Design review of the part built by this model. Coordinates are the model's own, in mm. Face numbers are marked on the shaded views. A direction names the side the tool comes from. Give positions to 0.01 mm unless a question says otherwise; leave off trailing zeros. Loops run counter-clockwise (first coordinate to the right, second up) from the corner with the lowest first, then second, coordinate; pieces in that order, holes last.
Autodesk Inventor part; units mm, degrees
ref_plane "YZ Plane" through (0, 0, 0) normal (1, 0, 0) x (0, 1, 0)
ref_plane "XZ Plane" through (0, 0, 0) normal (0, 1, 0) x (-1, 0, 0)
ref_plane "XY Plane" through (0, 0, 0) normal (0, 0, 1) x (1, 0, 0)
sketch "Sketch8" plane through (0, 0, 0) normal (0, 1, 0) x (-1, 0, 0)
  line L0 (-13.5, -17.5) -> (13.5, -17.5)
  line L1 (13.5, -17.5) -> (13.5, 17.5)
  line L2 (13.5, 17.5) -> (-13.5, 17.5)
  line L3 (-13.5, 17.5) -> (-13.5, -17.5)
  line L4 (-13.5, -17.5) -> (13.5, 17.5) construction
  line L5 (13.5, -17.5) -> (-13.5, 17.5) construction
  circle A0 centre (10, -7.5) radius 1.6
  circle A1 centre (10, 7.5) radius 1.6
  circle A2 centre (-10, 7.5) radius 1.6
  circle A3 centre (-10, -7.5) radius 1.6
  point P0 (0, 0)
  dimension "d38" = 35
  dimension "d39" = 27
  dimension "d40" = 20
  dimension "d41" = 15
  dimension "d42" = 7.5
  dimension "d43" = 10
  dimension "d44" = 3.2
extrude "Extrusion7" add sketch "Sketch8" against normal blind 3
sketch "Sketch14" plane through (0, 0, 0) normal (0, 1, 0) x (1, 0, 0)
  line L0 (-13.5, 17.5) -> (-13.5, -17.5)
  line L1 (-13.5, -17.5) -> (13.5, -17.5)
  line L2 (13.5, -17.5) -> (13.5, 17.5)
  line L3 (13.5, 17.5) -> (-13.5, 17.5)
  circle A0 centre (-10, 7.5) radius 1.6
  circle A1 centre (-10, -7.5) radius 1.6
  circle A2 centre (10, -7.5) radius 1.6
  circle A3 centre (10, 7.5) radius 1.6
  line L4 (13.5, -17.5) -> (13.5, 17.5)
  line L5 (13.5, 4.5) -> (7.5, 4.5)
  line L6 (7.5, 4.5) -> (7.5, -4.5)
  line L7 (7.5, -4.5) -> (13.5, -4.5)
  line L8 (13.5, -4.5) -> (13.5, 4.5)
  point P0 (0, 0)
  dimension "d79" = 7.5
  dimension "d80" = 3
  dimension "d81" = 3
extrude "Extrusion12" add sketch "Sketch14" along normal blind 22.3 contours L2 L7 L6 L5
sketch "Sketch15" plane through (13.5, -3, 17.5) normal (1, 0, 0) x (0, 0, -1)
  line L0 (0, 3) -> (13, 3)
  line L1 (0, 3) -> (0, 0)
  line L2 (35, 0) -> (0, 0)
  line L3 (35, 3) -> (35, 0)
  line L4 (22, 3) -> (35, 3)
  line L5 (22, 3) -> (22, 25.3)
  line L6 (13, 25.3) -> (22, 25.3)
  line L7 (13, 3) -> (13, 25.3)
  line L8 (35, 3) -> (35, 0)
  line L9 (35, 0) -> (41.8017, 14.6399)
  circle A0 centre (35, 17.8) radius 2.6
  circle A1 centre (35, 17.8) radius 7.5
  circle A2 centre (0, 17.8) radius 2.6
  circle A3 centre (0, 17.8) radius 7.5
  line L10 (-275, -9) -> (225, -9)
  line L11 (0, 0) -> (-6.8017, 14.6399)
  line L12 (0, 25.3) -> (35, 25.3)
  point P0 (17.5, 3)
  point P1 (13, 25.3)
  point P2 (22, 25.3)
  dimension "d84" = 5.2
  dimension "d85" = 35
  dimension "d86" = 17.5
  dimension "d87" = 26.8
  dimension "d88" = 15
extrude "Extrusion13" add sketch "Sketch15" against normal blind 3 contours L1 L11 A3 L12 L7 L0 | L3 L4 L5 L12 A1 L9 | A3 | A1
sketch "Sketch16" plane through (10.5, -3, 17.5) normal (-1, 0, 0) x (0, 0, 1)
  arc A0 (-35, 25.3) -> (-41.8017, 14.6399) centre (-35, 17.8) ccw
  line L0 (-41.8017, 14.6399) -> (-35, 0)
  line L1 (-35, 3) -> (-35, 0)
  line L2 (-26.5199, 3) -> (-35, 3)
  line L3 (-26.5199, 3) -> (-23.4801, 3)
  line L4 (-22, 3) -> (-23.4801, 3)
  line L5 (-22, 25.3) -> (-22, 3)
  line L6 (-22, 25.3) -> (-35, 25.3)
  circle A1 centre (-35, 17.8) radius 2.6
  arc A2 (6.8017, 14.6399) -> (0, 25.3) centre (0, 17.8) ccw
  line L7 (0, 25.3) -> (-13, 25.3)
  line L8 (-13, 3) -> (-13, 25.3)
  line L9 (-11.5199, 3) -> (-13, 3)
  line L10 (-11.5199, 3) -> (-8.4801, 3)
  line L11 (0, 3) -> (-8.4801, 3)
  line L12 (0, 0) -> (0, 3)
  line L13 (0, 0) -> (6.8017, 14.6399)
  circle A3 centre (0, 17.8) radius 2.6
  line L14 (-22, 3) -> (-29, 3)
  line L15 (-29, 3) -> (-29, 13)
  line L16 (-29, 13) -> (-22, 13)
  line L17 (-22, 13) -> (-22, 3)
  line L18 (-11.5199, 3) -> (-13, 3)
  line L19 (-13, 3) -> (-6, 3)
  line L20 (-6, 3) -> (-6, 13)
  line L21 (-6, 13) -> (-13, 13)
  line L22 (-13, 13) -> (-13, 3)
  line L23 (-23.4, 0) -> (-26.6, 0)
  line L24 (-26.6, 3) -> (-23.4, 3)
  line L25 (-8.4, 0) -> (-11.6, 0)
  line L26 (-11.6, 3) -> (-8.4, 3)
  point P0 (-17.5, 3)
  point P1 (-10, 0)
  point P2 (-6, 3)
  dimension "d91" = 7
  dimension "d92" = 3
  dimension "d93" = 10
extrude "Extrusion14" cut sketch "Sketch16" against normal blind 22.3 contours L5 L4 L3 L2 L15 L16 | L21 L20 L11 L10 L9 L8
sketch "Sketch17" plane through (10.5, -3, 17.5) normal (-1, 0, 0) x (0, 0, 1)
  circle A0 centre (-35, 17.8) radius 2.6
  line L0 (-29, 3) -> (-29, 13)
  line L1 (-29, 13) -> (-22, 13)
  line L2 (-22, 25.3) -> (-22, 13)
  line L3 (-22, 25.3) -> (-35, 25.3)
  arc A1 (-35, 25.3) -> (-41.8017, 14.6399) centre (-35, 17.8) ccw
  line L4 (-41.8017, 14.6399) -> (-35, 0)
  line L5 (-35, 3) -> (-35, 0)
  line L6 (-29, 3) -> (-35, 3)
  circle A2 centre (0, 17.8) radius 2.6
  line L7 (-13, 13) -> (-6, 13)
  line L8 (-6, 13) -> (-6, 3)
  line L9 (0, 3) -> (-6, 3)
  line L10 (0, 0) -> (0, 3)
  line L11 (0, 0) -> (6.8017, 14.6399)
  arc A3 (6.8017, 14.6399) -> (0, 25.3) centre (0, 17.8) ccw
  line L12 (0, 25.3) -> (-13, 25.3)
  line L13 (-13, 13) -> (-13, 25.3)
  line L14 (-13, 13) -> (-10, 25.3)
  line L15 (-22, 13) -> (-25, 25.3)
  line L16 (-35, 25.3) -> (0, 25.3)
  point P0 (-17.5, 3)
  dimension "d96" = 15
extrude "Extrusion15" add sketch "Sketch17" along normal up to surface (3 mm away) contours L12 L14 L13 | L15 L3 L2
fillet "Fillet2" radius 2 2 edges at (9, 22.3, -7.5) (9, 22.3, 7.5)
mirror "Mirror1" about plane through (0, 0, 0) normal (1, 0, 0) of "Extrusion12", "Extrusion13", "Extrusion14", "Extrusion15", "Fillet2"
chamfer "Chamfer1" distance 5 angle 45 4 edges at (-10.5, 0, 14.5) (-10.5, 0, -14.5) (10.5, 0, 14.5) (10.5, 0, -14.5)
sketch "Sketch18" plane through (-13.5, 22.3, -17.5) normal (-1, 0, 0) x (0, 0, 1)
  line L0 (13, -22.3) -> (6, -22.3)
  line L1 (6, -22.3) -> (6, -12.3)
  line L2 (6, -12.3) -> (13, -12.3)
  line L3 (13, -12.3) -> (13, -22.3)
  line L4 (29, -22.3) -> (22, -22.3)
  line L5 (22, -22.3) -> (22, -12.3)
  line L6 (22, -12.3) -> (29, -12.3)
  line L7 (29, -12.3) -> (29, -22.3)
  circle A0 centre (0, -7.5) radius 2.6
  circle A1 centre (35, -7.5) radius 2.6
  line L8 (41.8017, -10.6601) -> (35, -25.3)
  arc A2 (41.8017, -10.6601) -> (35, 0) centre (35, -7.5) ccw
  line L9 (0, 0) -> (35, 0)
  arc A3 (0, 0) -> (-6.8017, -10.6601) centre (0, -7.5) ccw
  line L10 (0, -25.3) -> (-6.8017, -10.6601)
  line L11 (35, -25.3) -> (0, -25.3)
  point P0 (17.5, -22.3)
  point P1 (17.5, -7)
  point P2 (17.5, -15.3)
  dimension "d103" = 7
  dimension "d104" = 10
hole "Hole3" at (-13.5, 15.3, 0) at (-13.5, 7, 0) direction (1, 0, 0) diameter 3.6 end through all
sketch "Sketch19" plane through (13.5, 22.3, 17.5) normal (1, 0, 0) x (0, 0, -1)
  circle A0 centre (17.5, -15.3) radius 1.8
  circle A1 centre (17.5, -7) radius 1.8
  circle A2 centre (17.5, -15.3) radius 3.25
  circle A3 centre (17.5, -7) radius 3.25
  point P0 (17.5, -22.3)
  dimension "d112" = 6.5
extrude "Extrusion16" cut sketch "Sketch19" against normal blind 3 contours A0 | A1 | A2 | A3
sketch "Sketch20" plane through (-13.5, 22.3, -17.5) normal (-1, 0, 0) x (0, 0, 1)
  circle A0 centre (17.5, -15.3) radius 3.25
  circle A1 centre (17.5, -7) radius 3.25
  point P0 (17.5, -22.3)
extrude "Extrusion17" cut sketch "Sketch20" against normal blind 3
equation "\"d81\" = d80"
properties part number "Y Axis Gantry Baseblock (CNC)" material "ABS Plastic"
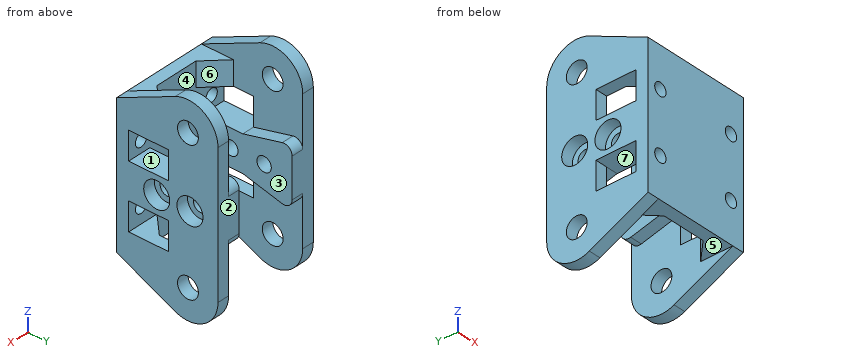
Q1. Take a section at C-C (y = 20.75). Give the boundary of the cut face in (x, z).
Results:
outline: (-13.5, -22.07) - (-10.5, -22.07) - (-10.5, -6.9) - (-7.5, -6.9) - (-7.5, 6.9) - (-10.5, 6.9) - (-10.5, 22.07) - (-13.5, 22.07) - close; (7.5, -6.9) - (10.5, -6.9) - (10.5, -22.07) - (13.5, -22.07) - (13.5, 22.07) - (10.5, 22.07) - (10.5, 6.9) - (7.5, 6.9) - close
Q2. Insertion check: pin 1 (5 mm diameter, centred on x = -12, y = 3.5, fed in from +Z); pin 2 (5 mm diameter, centred on y = 7.5, z = 0, fed in from +X); pin 3 (12 mm diameter, centred on x = 7, z = 18, fed in from +Y); pin 4 (4.5 mm diameter, centred on y = 7, z = 0, fed in from -X). Each pin has a flat end and moves straight along its axis. Give the tip position at first contact, or say it passes through.
Results:
pin 1: stops at z = 21.68
pin 2: stops at x = 10.5
pin 3: stops at y = 22.3
pin 4: stops at x = -10.5
Q3. Wall thickness on line 1 (Z direction, x = -10, y = -0.25); line 2 (X direction, y = -2.1, z = -7.5); line 3 (Y direction, x = -12.9, z = 0): over which ranges is each line inside the solid? List them lowest first.
Results:
line 1: z = -17.5 to -9.1, -5.9 to 5.9, 9.1 to 17.5
line 2: x = -13.5 to -11.6, -8.4 to 8.4, 11.6 to 13.5
line 3: y = -3 to 3.75, 10.25 to 12.05, 18.55 to 22.3
Q4. Tool access review of the marked faces 4, 5, 6 and 7: name each direction out of +Z, -Z, +X, -X, +Y, -Y from which nothing blocks a thin tool from reaching the whole face with its end or side.
Results:
face 4: none
face 5: -Z, +Y, -Y
face 6: +Z, +Y
face 7: +X, -X
Q5. Take a section at B-B (x = -10). Give the boundary of the cut face in (y, z), plus the area to 3 significant figures.
Results:
outline: (-3, -17.5) - (4.5, -17.5) - (4.5, -11.5) - (0, -11.5) - (0, -9.1) - (-3, -9.1) - close; (-3, -5.9) - (0, -5.9) - (0, -4.5) - (10, -4.5) - (19.83, -6.9) arc R2 ccw to (22.3, -4.95) - (22.3, 4.95) arc R2 ccw to (19.83, 6.9) - (10, 4.5) - (0, 4.5) - (0, 5.9) - (-3, 5.9) - close; (-3, 9.1) - (0, 9.1) - (0, 11.5) - (4.5, 11.5) - (4.5, 17.5) - (-3, 17.5) - close; hole circle Ø3.6 at (7, 0); hole circle Ø3.6 at (15.3, 0)
area: 354 mm2
Q6. Draft analysis for pull direction Y (two halves, no side actions). For the marked faces 1, 2 and 3, state which applies: pulls with the +Y half, pulls with the -Y half, needs draft (parallel to the pull), parting line crosses it, or undercut.
Results:
face 1: undercut
face 2: pulls with the +Y half
face 3: needs draft
Q7. Take a section at D-D (x = 6.75). Give the boundary of the cut face in (y, z), plus the area to 3 significant figures.
Results:
outline: (-3, -17.5) - (1.25, -17.5) - (1.25, -11.5) - (0, -11.5) - (0, 11.5) - (1.25, 11.5) - (1.25, 17.5) - (-3, 17.5) - close
area: 120 mm2
Q8. Take a section at A-A (z = 7.5). Give the boundary of the cut face in (x, y), plus the area to 3 significant figures.
Results:
outline: (-13.5, -3) - (-11.6, -3) - (-11.6, 0) - (-13.5, 0) - close; (-13.5, 10) - (-10.5, 10) - (-10.5, 22.3) - (-13.5, 22.3) - close; (-8.4, -3) - (8.4, -3) - (8.4, 0) - (-8.4, 0) - close; (10.5, 10) - (13.5, 10) - (13.5, 22.3) - (10.5, 22.3) - close; (11.6, -3) - (13.5, -3) - (13.5, 0) - (11.6, 0) - close
area: 136 mm2
